Build history of the part. All positions in model axes, mm. Round coordinates to 2 decimals unless told otherwise and drop trailing zeros. Write each loop counter-clockwise with the first axis right and the second up, starting at its lowest first coordinate (ties: lowest second). Pieces come first, ordered by that corner, then holes. Notation, with made-up numbers: M 79,-15 L 110,-15 A15 cw 110,-10 Z; hole C -10,75.5 d1. An arc over 180 degrees is marked long. Write item = value, one per line. Start each with the question number.
Q1. Band-saw the part on C-C on y = 61. Write the cut outline in (x, z), plus the area to 3 significant figures.
Q2. Band-saw the part on B-B on x = 2.55. Write the cut outline in (y, z) (3 decimals), plus the area to 3 significant figures.
Q3. Probe L1, parallel to Y at x = 1.75, z = 0; L2, parallel to Z at x = 0.9, y = 266; L3, parallel to Y at x = 1.65, z = 8. List the from-to ranges inside material, lowest first.
Q4. Drop a flat-ended pin along its axis: P1, Ø1.5, axis at x = 4, y = 113, coming from the -Z side. Give the stop position or say it passes through.
Q5. Band-saw the part on A-A on z = 0. Write the cut outline in (x, y), plus the area to 3 significant figures.
Q6. Band-saw the part on D-D on y = 170. Write the cut outline in (x, z), plus the area to 3 significant figures.
```python
from build123d import *

# Parameters (mm, degrees)
EXTRUDE_1_DEPTH     = 5
SKETCH_2_R          = 2
SKETCH_2_R_2        = 4
CUT_EXTRUDE_1_DEPTH = 293.792434527


with BuildPart() as part:
    # 草图1 → 凸台-拉伸1 (new body)
    with BuildSketch(Plane(origin=(0, 0, 0), x_dir=(0, 0, -1), z_dir=(1, 0, 0))):
        with BuildLine():
            ThreePointArc((-12.5, 0), (0, -12.5), (12.5, 0))
            ThreePointArc((12.5, 0), (33.57319831, 124.194448186), (40, 250))
            ThreePointArc((40, 250), (0, 290), (-40, 250))
            ThreePointArc((-40, 250), (-33.57319831, 124.194448186), (-12.5, 0))
        make_face()
    extrude(amount=EXTRUDE_1_DEPTH)

    # 草图2 → 切除-拉伸1 (cut, through all)
    with BuildSketch(Plane.ZY):
        with Locations((17.25, 250)):
            Circle(SKETCH_2_R)
        with Locations((8.625, 235.061061785)):
            Circle(SKETCH_2_R)
        with Locations((-8.625, 235.061061785)):
            Circle(SKETCH_2_R)
        with Locations((-17.25, 250)):
            Circle(SKETCH_2_R)
        with Locations((-8.625, 264.938938215)):
            Circle(SKETCH_2_R)
        with Locations((8.625, 264.938938215)):
            Circle(SKETCH_2_R)
        with Locations((0, 250)):
            Circle(SKETCH_2_R_2)
    extrude(amount=-CUT_EXTRUDE_1_DEPTH, mode=Mode.SUBTRACT)


solid = part.part
```
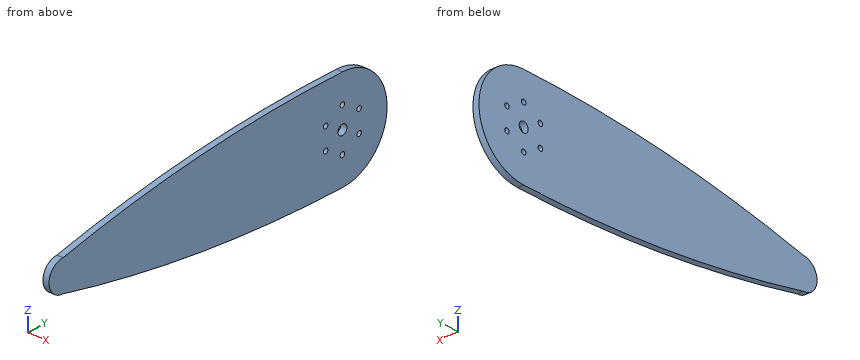
Conclusion:
q1.outline = M 0,-24.72 L 5,-24.72 L 5,24.72 L 0,24.72 Z
q1.area = 247 mm^2
q2.outline = M 0,-12.5 A1076.934 ccw 250,-40 A40 ccw 250,40 A1076.934 ccw 0,12.5 A12.5 ccw Z; hole C 235.061,-8.625 d4; hole C 235.061,8.625 d4; hole C 250,0 d8; hole C 250,-17.25 d4; hole C 250,17.25 d4; hole C 264.939,-8.625 d4; hole C 264.939,8.625 d4
q2.area = 18,200 mm^2
q3.L1 = -12.5 to 246, 254 to 290
q3.L2 = -36.66 to -10.32, -6.93 to 6.93, 10.32 to 36.66
q3.L3 = -9.6 to 233.16, 236.96 to 263.04, 266.84 to 289.19
q4.P1 = -32.37
q5.outline = M 0,-12.5 L 5,-12.5 L 5,246 L 0,246 Z; M 0,254 L 5,254 L 5,290 L 0,290 Z
q5.area = 1,470 mm^2
q6.outline = M 0,-37.62 L 5,-37.62 L 5,37.62 L 0,37.62 Z
q6.area = 376 mm^2
